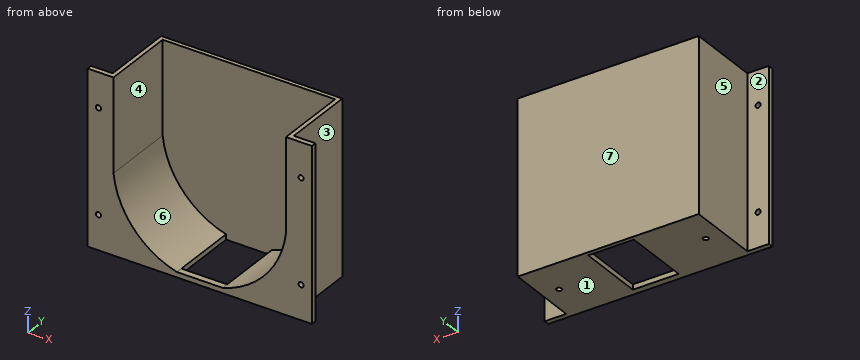
```python
from build123d import *

# Parameters (mm, degrees)
SKETCH1_W           = 105
SKETCH1_H           = 75
SKETCH1_W_2         = 100
SKETCH1_H_2         = 70
BOSS_EXTRUDE1_DEPTH = 100
SKETCH1_2_W         = 105
SKETCH1_2_H         = 75
BOSS_EXTRUDE2_DEPTH = 3
BOSS_EXTRUDE3_DEPTH = 73
CUT_EXTRUDE3_START  = -21.5
CUT_EXTRUDE3_DEPTH  = 21.5
CUT_EXTRUDE4_START  = -30
CUT_EXTRUDE4_DEPTH  = 30
SKETCH7_W           = 26.515577751
SKETCH7_H           = 38.587429438
CUT_EXTRUDE5_DEPTH  = 71
SKETCH8_W           = 12.5
SKETCH8_H           = 100
SKETCH8_R           = 1.5
BOSS_EXTRUDE4_DEPTH = 3
SKETCH9_R           = 1.5
CUT_EXTRUDE6_DEPTH  = 6


with BuildPart() as part:
    # Sketch1 → Boss-Extrude1 (new body)
    with BuildSketch(Plane.XY):
        with Locations((-17.926459532, -39.040517308)):
            Rectangle(SKETCH1_W, SKETCH1_H)
        with Locations((-17.926459532, -39.040517308)):
            Rectangle(SKETCH1_W_2, SKETCH1_H_2, mode=Mode.SUBTRACT)
    extrude(amount=BOSS_EXTRUDE1_DEPTH)

    # Sketch1_2 → Boss-Extrude2 (add)
    with BuildSketch(Plane.XY):
        with Locations((-17.926459532, -39.040517308)):
            Rectangle(SKETCH1_2_W, SKETCH1_2_H)
    extrude(amount=BOSS_EXTRUDE2_DEPTH)

    # Sketch4 → Boss-Extrude3 (add)
    with BuildSketch(Plane(origin=(0, -1.540517308, 0), x_dir=(1, 0, 0), z_dir=(0, 1, 0))):
        with BuildLine():
            Line((-67.926459532, -3), (-67.926459532, -46.206705574))
            ThreePointArc((-67.926459532, -46.206705574), (-56.229094102, -18.928123314), (-31.184248407, -3))
            Line((-31.184248407, -3), (-67.926459532, -3))
        make_face()
        with BuildLine():
            Line((32.352949433, -3), (-4.668670656, -3))
            ThreePointArc((-4.668670656, -3), (22.039856002, -20.992417524), (32.352949433, -51.5))
            Line((32.352949433, -51.5), (32.352949433, -3))
        make_face()
    extrude(amount=-BOSS_EXTRUDE3_DEPTH)

    # Sketch5 → Cut-Extrude3 (cut)
    with BuildSketch(Plane.XZ.offset(76.540517308).offset(CUT_EXTRUDE3_START)):
        with BuildLine():
            Line((31.63486206, 100), (-67.926459532, 100))
            Line((-67.926459532, 100), (-67.926459532, 46.206705574))
            ThreePointArc((-67.926459532, 46.206705574), (-56.361491054, 19.084458701), (-31.579033768, 3.109647836))
            Line((-31.579033768, 3.109647836), (-4.273885295, 3.109647836))
            ThreePointArc((-4.273885295, 3.109647836), (19.456191853, 17.876253312), (31.63486206, 43.032747318))
            Line((31.63486206, 43.032747318), (31.63486206, 100))
        make_face()
    extrude(amount=CUT_EXTRUDE3_DEPTH, mode=Mode.SUBTRACT)

    # Sketch6 → Cut-Extrude4 (cut)
    with BuildSketch(Plane.XZ.offset(76.540517308).offset(CUT_EXTRUDE4_START)):
        with BuildLine():
            Line((-67.926459532, 46.206705574), (-67.926459532, 100))
            Line((-67.926459532, 100), (-70.426459532, 100))
            Line((-70.426459532, 100), (-70.426459532, 0))
            Line((-70.426459532, 0), (34.573540468, 0))
            Line((34.573540468, 0), (34.573540468, 100))
            Line((34.573540468, 100), (31.63486206, 100))
            Line((31.63486206, 100), (31.63486206, 43.032747318))
            ThreePointArc((31.63486206, 43.032747318), (19.456191853, 17.876253312), (-4.273885295, 3.109647836))
            Line((-4.273885295, 3.109647836), (-31.579033768, 3.109647836))
            ThreePointArc((-31.579033768, 3.109647836), (-56.361491054, 19.084458701), (-67.926459532, 46.206705574))
        make_face()
    extrude(amount=CUT_EXTRUDE4_DEPTH, mode=Mode.SUBTRACT)

    # Sketch7 → Cut-Extrude5 (cut)
    with BuildSketch(Plane.XY.offset(3)):
        with Locations((-17.926459532, -23.334232027)):
            Rectangle(SKETCH7_W, SKETCH7_H)
    extrude(amount=-CUT_EXTRUDE5_DEPTH, mode=Mode.SUBTRACT)

    # Sketch8 → Boss-Extrude4 (add)
    # profile 1 of 2: a face of its own
    with BuildSketch(Plane.XZ.offset(46.540517308)):
        with Locations((-76.676459532, 50)):
            Rectangle(SKETCH8_W, SKETCH8_H)
        with Locations(Location((-76.676459532, 20, 0), (0, 0, 270))):
            Circle(SKETCH8_R, mode=Mode.SUBTRACT)
        with Locations(Location((-76.676459532, 80, 0), (0, 0, 270))):
            Circle(SKETCH8_R, mode=Mode.SUBTRACT)
    # profile 2 of 2: a face of its own
    with BuildSketch(Plane.XZ.offset(46.540517308)):
        with Locations((40.823540468, 50)):
            Rectangle(SKETCH8_W, SKETCH8_H)
        with Locations(Location((40.823540468, 20, 0), (0, 0, 270))):
            Circle(SKETCH8_R, mode=Mode.SUBTRACT)
        with Locations(Location((40.823540468, 80, 0), (0, 0, 270))):
            Circle(SKETCH8_R, mode=Mode.SUBTRACT)
    extrude(amount=-BOSS_EXTRUDE4_DEPTH)

    # Sketch9 → Cut-Extrude6 (cut)
    with BuildSketch(Plane(origin=(0, 0, 0), x_dir=(-1, 0, 0), z_dir=(0, 0, -1))):
        with Locations((-24.573540468, -22.540517308)):
            Circle(SKETCH9_R)
        with Locations((60.426459532, -22.540517308)):
            Circle(SKETCH9_R)
    extrude(amount=-CUT_EXTRUDE6_DEPTH, mode=Mode.SUBTRACT)


solid = part.part
```
Here's how the part is built. I have some questions about the finished solid (model axes, mm). Face numbers are marked on the shaded views. A direction names the side the tool comes from. Coordinates: 2 decimals unless noted, no trailing zeros. Order: outer loops, then holes, each group sorted by start corner. A loop starts at its lowest first (then second) coordinate and runs counter-clockwise, first axis right, second up. Notation, with made-up numbers: (-24, 19) -> (12, 19) arc R10 ccw to (12, 38) -> close; hole circle Ø10 at (33.25, 32.25). An arc over 180 degrees is marked (long way). Return JSON: item names as keys, results as strings.
1) If we section it at D-D on z = 67: List the corners of the cut face in (x, y) for me.
Conclusion:
{"outline": "(-82.93, -46.54) -> (-67.93, -46.54) -> (-67.93, -4.04) -> (32.07, -4.04) -> (32.07, -46.54) -> (47.07, -46.54) -> (47.07, -43.54) -> (34.57, -43.54) -> (34.57, -1.54) -> (-70.43, -1.54) -> (-70.43, -43.54) -> (-82.93, -43.54) -> close"}
2) Thinking about a two-plate mould opening in X: for the marked faces 5, 6 and 7, which applies, +X half, -X half, draft (parallel to the pull), parting line (faces both ways), or undercut?
Conclusion:
{"face 5": "-X half", "face 6": "undercut", "face 7": "draft"}
3) On a 3-axis mill with a long thin cutter (end or side, diameter ignored), from which of +Z, -Z, +X, -X, +Y, -Y can I reach the whole of each face in a straight line? I mean the marked faces 1, 2, 3 and 4. Say none if no direction works.
Conclusion:
{"face 1": "-Z, +X, -X, +Y, -Y", "face 2": "+Z, -Z, -X, +Y", "face 3": "+Z, -Z, +X, +Y", "face 4": "+Z, -Y"}
4) If we section it at A-A on y = -38.5: List the corners of the cut face in (x, z) for me.
Conclusion:
{"outline": "(-70.43, 0) -> (-31.18, 0) -> (-31.18, 3) arc R50.28 cw to (-67.93, 46.21) -> (-67.93, 100) -> (-70.43, 100) -> close; (-4.67, 0) -> (34.57, 0) -> (34.57, 100) -> (32.07, 100) -> (32.07, 46.21) arc R50.28 cw to (-4.67, 3) -> close"}
5) If we section it at C-C on z = 80: List the corners of the cut face in (x, y) for me.
Conclusion:
{"outline": "(-82.93, -46.54) -> (-78.18, -46.54) -> (-78.18, -43.54) -> (-82.93, -43.54) -> close; (-75.18, -46.54) -> (-67.93, -46.54) -> (-67.93, -4.04) -> (32.07, -4.04) -> (32.07, -46.54) -> (39.32, -46.54) -> (39.32, -43.54) -> (34.57, -43.54) -> (34.57, -1.54) -> (-70.43, -1.54) -> (-70.43, -43.54) -> (-75.18, -43.54) -> close; (42.32, -46.54) -> (47.07, -46.54) -> (47.07, -43.54) -> (42.32, -43.54) -> close"}
6) I'm going to push flat-ended pins straight in: P1, Ø4, axis at x = 41.5, z = 53, coming from the +Y side; P2, Ø1.5, axis at x = 24.5, y = -22.5, coming from the -Z side; P3, Ø2, axis at y = -37, z = 48.5, coming from the +X side. Where does each tip first touch, or does it pass through?
Conclusion:
{"P1": "stops at y = -43.54", "P2": "stops at z = 6", "P3": "stops at x = 34.57"}
7) If we section it at B-B on x = -10: List the corners of the cut face in (y, z) for me.
Conclusion:
{"outline": "(-46.54, 0) -> (-42.63, 0) -> (-42.63, 3) -> (-46.54, 3) -> close; (-4.04, 0) -> (-1.54, 0) -> (-1.54, 100) -> (-4.04, 100) -> close"}
8) If I drill on probe 1 along X at (y, z) = (-45.6, 80); probe 2 along X at (y, z) = (-38.5, 78.5); probe 3 along X at (y, z) = (-45, 20), over which ranges is the centre line in solid material (lowest first)?
Conclusion:
{"probe 1": "x = -82.93 to -78.18, -75.18 to -67.93, 32.07 to 39.32, 42.32 to 47.07", "probe 2": "x = -70.43 to -67.93, 32.07 to 34.57", "probe 3": "x = -82.93 to -78.18, -75.18 to -57.12, 21.26 to 39.32, 42.32 to 47.07"}
